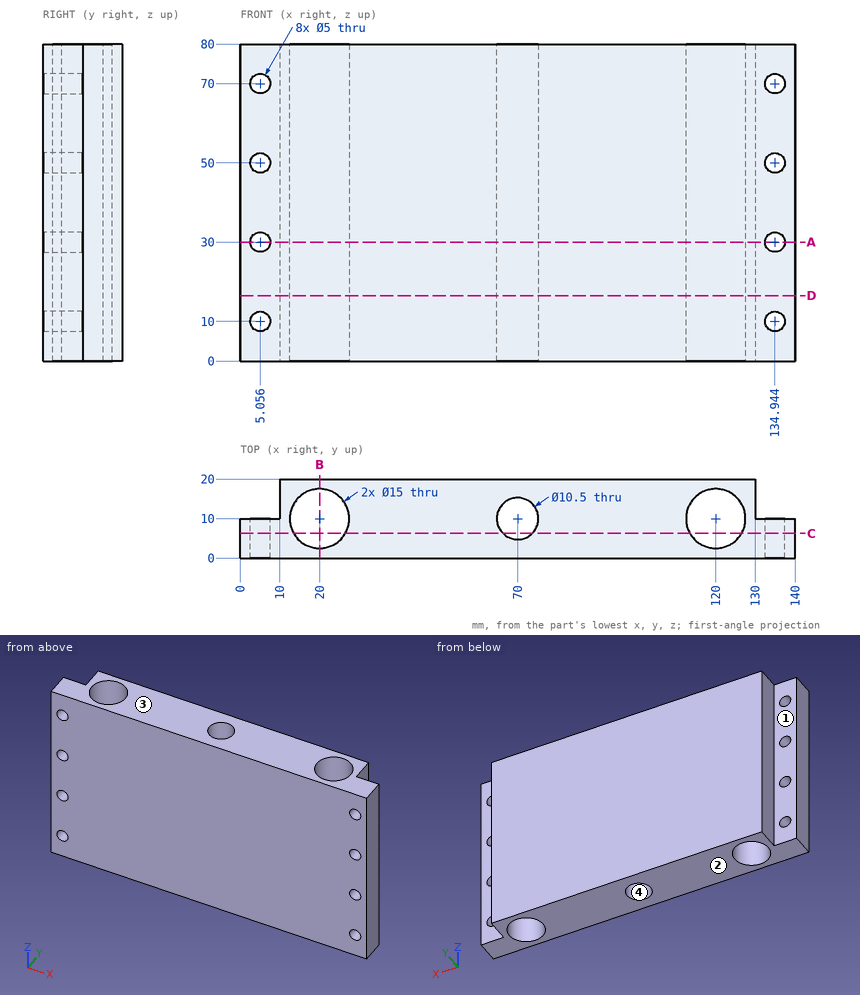
Here's the drawing with two shaded views (mm, measured from the low corner). I have some questions. A direction names the side the tool comes from. Coordinates: 2 decimals unless noted, no trailing zeros. Write each loop counter-clockwise with the first axis right and the second up, starting at its lowest first coordinate (ties: lowest second). Pieces come first, ordered by that corner, then holes. Notation, with made-up numbers: M 72.25,47 L 94.25,47 A26 cw 94.25,76 Z; hole C 22.5,24.5 d5. An arc over 180 degrees is marked long. Answer as CSV lines item,"result".
Item 1: I'm going to push flat-ended pins straight in: P1, Ø6, axis at x = 134.94, z = 70, coming from the +Y side; P2, Ø5, axis at y = 14, z = 57.5, coming from the -X side; P3, Ø4.5, axis at x = 5.06, z = 70, coming from the +Y side; P4, Ø1, axis at y = 13.5, z = 17, coming from the +X side. Where does each tip first touch, or does it pass through?
Geometry results:
P1,"stops at y = 10"
P2,"stops at x = 10"
P3,"passes through"
P4,"stops at x = 130"
Item 2: Please list where these lines run through material, in increasing order: line 1 along X through (y, z) = (16, 74); line 2 along X through (y, z) = (2, 30); line 3 along X through (y, z) = (11, 56).
Geometry results:
line 1,"x = 10 to 15.5, 24.5 to 115.5, 124.5 to 130"
line 2,"x = 0 to 2.56, 7.56 to 132.44, 137.44 to 140"
line 3,"x = 10 to 12.57, 27.43 to 64.85, 75.15 to 112.57, 127.43 to 130"
Item 3: On a 3-axis mill with a long thin cutter (end or side, diameter ignored), from which of +Z, -Z, +X, -X, +Y, -Y can I reach the whole of each face in a straight line? I mean the marked faces 1 and 2. Say none if no direction works.
Geometry results:
face 1,"+Z, -Z, -X, +Y"
face 2,"-Z, +X, -X, +Y, -Y"
Item 4: Imagine slicing it at C-C on y = 6.25. State how many separate pieces and enclosed holes the cut face has, plus the area to 3 significant figures.
Geometry results:
separate pieces,"4"
enclosed holes,"8"
area,"8,380 mm2"
Item 5: Imagine slicing it at D-D on z = 16.5. List the corners of the cut face in (x, y) for me, plus the area to 3 significant figures.
Geometry results:
outline,"M 0,0 L 140,0 L 140,10 L 130,10 L 130,20 L 10,20 L 10,10 L 0,10 Z; hole C 20,10 d15; hole C 70,10 d10.5; hole C 120,10 d15"
area,"2,160 mm2"
Item 6: Imagine slicing it at A-A on z = 30. List the corners of the cut face in (x, y) for me.
Geometry results:
outline,"M 0,0 L 2.56,0 L 2.56,10 L 0,10 Z; M 7.56,0 L 132.44,0 L 132.44,10 L 130,10 L 130,20 L 10,20 L 10,10 L 7.56,10 Z; M 137.44,0 L 140,0 L 140,10 L 137.44,10 Z; hole C 20,10 d15; hole C 70,10 d10.5; hole C 120,10 d15"
Item 7: We'd pull the mould along X, two halves only. Please class the marked faces 3 and 4: +X half, -X half, draft (parallel to the pull), parting line (faces both ways), or undercut.
Geometry results:
face 3,"draft"
face 4,"undercut"
Item 8: Imagine slicing it at B-B on x = 20. List the corners of the cut face in (y, z) for me, plus the area to 3 significant figures.
Geometry results:
outline,"M 0,0 L 2.5,0 L 2.5,80 L 0,80 Z; M 17.5,0 L 20,0 L 20,80 L 17.5,80 Z"
area,"400 mm2"
